Check sheet for the modelled part. Datum: model origin and axes. Units: mm. Face numbers are marked on the shaded views. A direction names the side the tool comes from. Round coordinates to 2 decimals unless told otherwise and drop trailing zeros. Loops run counter-clockwise (first coordinate to the right, second up) from the corner with the lowest first, then second, coordinate; pieces in that order, holes last. Notation, with made-up numbers: M 48.5,-12 L 82.5,-12 A6 ccw 82.5,-5 Z; hole C -36.75,11 d3. An arc over 180 degrees is marked long. Write item = value, one per line. Start each with the question number.
(1) Cross-section at A-A on x = 3.5. Record the boundary of the cut face in (y, z).
(2) Go/stop test with a flat-tipped pin: P1, Ø1.8, axis at x = 3.5, y = 12.5, coming from the -Z side. Record where the tip stops, or that it passes through.
(3) Cross-section at C-C on x = 5. Record the boundary of the cut face in (y, z), plus the area to 3 significant figures.
(4) Cross-section at D-D on z = -1.45. Record the boundary of the cut face in (x, y), plus the area to 3 significant figures.
(5) Scan lines: L1, parallel to Z at x = 0.25, y = 24.5; L2, parallel to Y at x = 4, z = 0.85; L3, parallel to Y at x = 2.5, z = 0.4. Record each from-to range of solid material in increasing order. Write a range as from..to.
(6) Set-up check for the marked faces 1 and 2: record each of +Z, -Z, +X, -X, +Y, -Y from which the full face is reachable in a straight line by a thin tool's end or side.
(7) Cross-section at B-B on y = 2.25. Record the boundary of the cut face in (x, z).
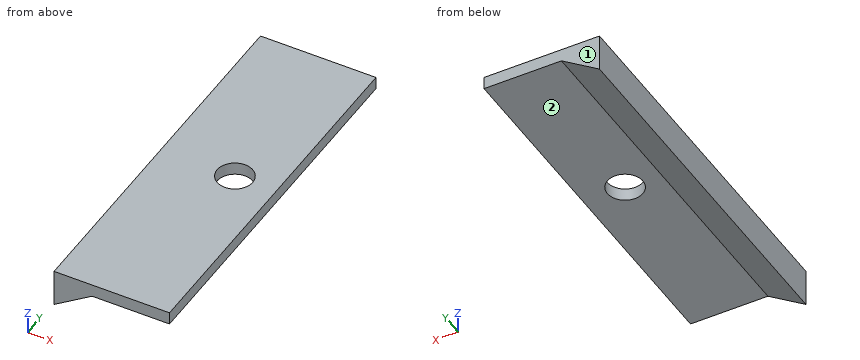
Autodesk Inventor part; units mm, degrees
ref_plane "YZ Plane" through (0, 0, 0) normal (1, 0, 0) x (0, 1, 0)
ref_plane "XZ Plane" through (0, 0, 0) normal (0, 1, 0) x (-1, 0, 0)
ref_plane "XY Plane" through (0, 0, 0) normal (0, 0, 1) x (1, 0, 0)
ref_plane "Work Plane1" through (0, 0, 0) normal (0, 0, 1) x (1, 0, 0)
sketch "Sketch1" plane through (0, 0, 0) normal (0, 0, 1) x (1, 0, 0)
  arc A0 (0, 9.6831) -> (0, 20.3535) centre (0, 15.0183) ccw
  line L0 (0, 0) -> (0, 9.6831)
  line L1 (6.1022, 0) -> (0, 0)
  line L2 (6.1022, 0) -> (6.1022, 29)
  line L3 (6.1022, 29) -> (0, 29)
  line L4 (0, 20.3535) -> (0, 29)
  line L5 (6.1022, 29) -> (-3, 29)
  line L6 (-3, 29) -> (-3, 0)
  line L7 (-3, 0) -> (6.1022, 0)
  line L8 (6.1022, 0) -> (6.1022, 29)
  circle A1 centre (2.8309, 15.0183) radius 1.4
  dimension "d0" = 3
extrude "Extrusion1" add sketch "Sketch1" along normal blind 1
sketch "Sketch2" plane through (-3, 0, 0) normal (0, -1, 0) x (1, 0, 0)
  line L0 (0, 0) -> (9.1022, 0)
  line L1 (9.1022, 0) -> (9.1022, 1)
  line L2 (0, 1) -> (9.1022, 1)
  line L3 (0, 0) -> (0, 1)
  line L4 (-3.1221, -0.6) -> (3.4779, -0.6)
  line L5 (9.1022, 0) -> (0, 0)
  line L6 (0, 0) -> (3, 0)
  line L7 (0, 0) -> (0, -1.9574)
  line L8 (0, -1.9574) -> (3, 0)
  point P0 (0, -0.6)
extrude "Extrusion2" add sketch "Sketch2" against normal up to surface (29 mm away) contours L0 L8 L4 L7 | L4 L8 L7
properties part number "cellSTORM_v5_chiptry_clamp"
Result:
q1.outline = M 0,0 L 13.79,0 L 13.79,1 L 0,1 Z; M 16.25,0 L 29,0 L 29,1 L 16.25,1 Z
q2.P1 = 0
q3.outline = M 0,0 L 29,0 L 29,1 L 0,1 Z
q3.area = 29.0 mm^2
q4.outline = M -3,0 L -2.22,0 L -2.22,29 L -3,29 Z
q4.area = 22.6 mm^2
q5.L1 = 0..1
q5.L2 = 0..14.25, 15.79..29
q5.L3 = 0..13.66, 16.38..29
q6.face_1 = +Z, -Z, +X, -X, +Y
q6.face_2 = -Z, +X, +Y, -Y
q7.outline = M -3,-1.96 L 0,0 L 6.1,0 L 6.1,1 L -3,1 Z
